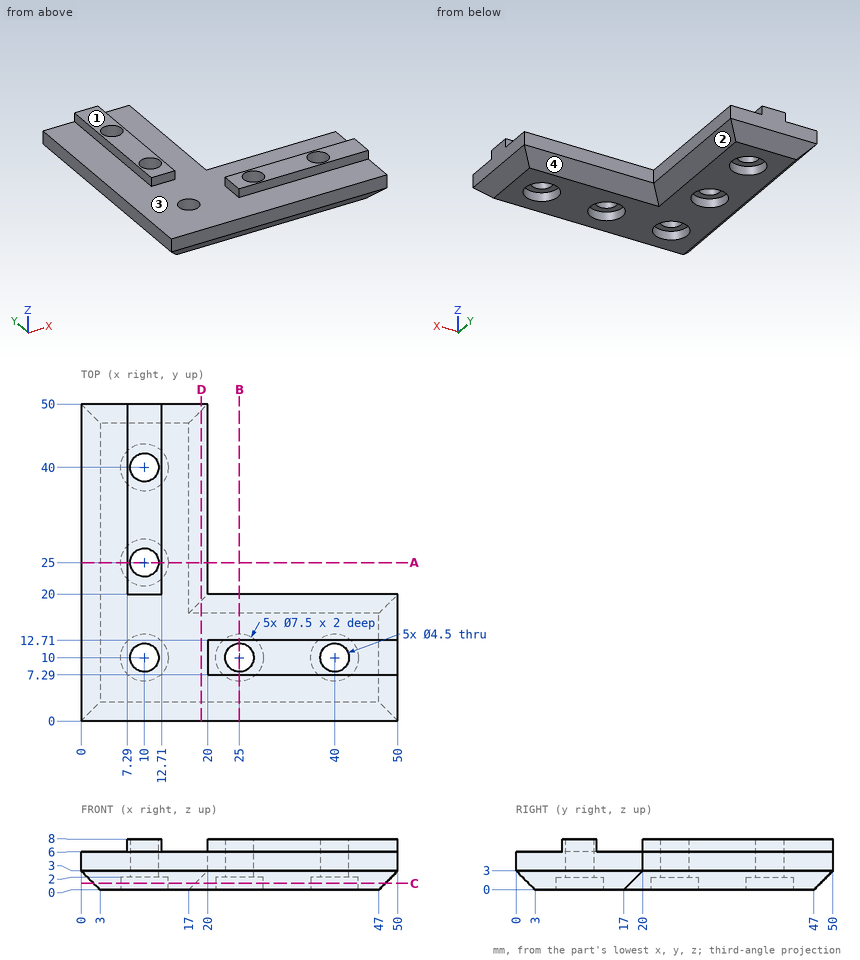
Geometry: see drawing. Coordinates: mm, zero at the bounding-box minimum. A direction names the side the tool comes from. Coordinates: 2 decimals unless noted, no trailing zeros. Order: outer loops, then holes, each group sorted by start corner. A loop starts at its lowest first (then second) coordinate and runs counter-clockwise, first axis right, second up. Notation, with made-up numbers: M -2.5,4 L 23.5,4 A14 cw 23.5,25 Z; hole C 78.5,-19 d4. An arc over 180 degrees is marked long. Write each question's results on one line, items separated by ' | '. Start each with the question number.
1) Contact query for flat-ended pins moving along their axis: pin 1 Ø2 at (y, z) = (11, 7.5) entering from -X; pin 2 Ø1.6 at (x, z) = (29, 6.5) entering from +Y; pin 3 Ø7 at (x, y) = (40, 10) entering from -Z. Output: stop coordinate, or through.
2) Line query: line 1 (Y direction, x = 10, z = 6.5); line 2 (Y direction, x = 10, z = 1.2); line 3 (X direction, y = 8, z = 7.75). Output: solid intervals per line, ascending. Write a range as from..to.
3) Section query A-A (y = 25). Return the cut outline in (x, z).
4) Section query D-D (x = 19). Return the cut outline in (y, z).
5) Draft query along Y for the marked faces 3 and 4. Return one class per face: released by +Y, released by -Y, zero draft, split by the parting line, or undercut.
6) Section query C-C (z = 1). Return the cut outline in (x, y).
7) Access query for the marked faces 1 and 2. Directions: +Z, -Z, +X, -X, +Y, -Y. A direction counts if a zero-diameter tool reaches every point of the face in a straight line with its end or side. Return the directions, or none.
Answers:
1) pin 1: stops at x = 20 | pin 2: stops at y = 20 | pin 3: stops at z = 2
2) line 1: y = 20..22.75, 27.25..37.75, 42.25..50 | line 2: y = 1.8..6.25, 13.75..21.25, 28.75..36.25, 43.75..48.2 | line 3: x = 20..23.97, 26.03..38.97, 41.03..50
3) outline: M 0,3 L 3,0 L 6.25,0 L 6.25,2 L 7.75,2 L 7.75,8 L 7.29,8 L 7.29,6 L 0,6 Z; M 12.25,2 L 13.75,2 L 13.75,0 L 17,0 L 20,3 L 20,6 L 12.71,6 L 12.71,8 L 12.25,8 Z
4) outline: M 0,3 L 3,0 L 17,0 L 19,2 L 49,2 L 50,3 L 50,6 L 0,6 Z
5) face 3: zero draft | face 4: released by +Y
6) outline: M 2,2 L 48,2 L 48,18 L 18,18 L 18,48 L 2,48 Z; hole C 10,10 d7.5; hole C 10,25 d7.5; hole C 10,40 d7.5; hole C 25,10 d7.5; hole C 40,10 d7.5
7) face 1: +Z, +X, -X, +Y, -Y | face 2: -Z, +X, +Y
